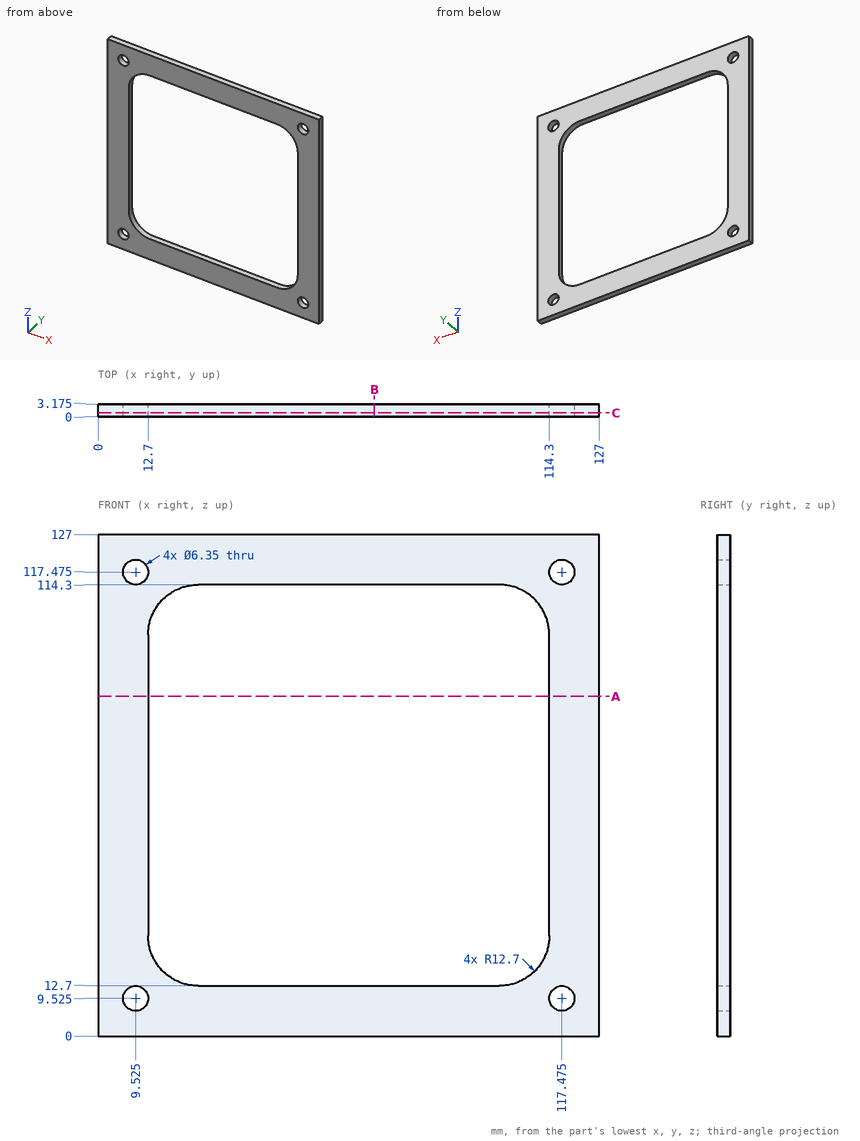
Geometry: see drawing. Coordinates: mm, zero at the bounding-box minimum. Coordinates: 2 decimals unless noted, no trailing zeros. Loops run counter-clockwise (first coordinate to the right, second up) from the corner with the lowest first, then second, coordinate; pieces in that order, holes last. Notation, with made-up numbers: M 6.25,45.25 L 12.25,45.25 A16 ccw 12.25,57.25 Z; hole C -13,54 d11. An arc over 180 degrees is marked long. Put each result on its own line as item: value. Start each with the question number.
1) Cut plane B-B on x = 70. Return the cut outline in (y, z) (3 decimals).
2) Cut plane C-C on y = 0.9. Return the cut outline in (x, z) (3 decimals).
3) Ray query, L1, parallel to Z at x = 36, y = 2.05; L2, parallel to Z at x = 118.5, y = 1.1. Return the intervals inside material, ascending. Write a range as from..to.
4) Cut plane A-A on z = 86. Return the cut outline in (x, y) (3 decimals), then the cut area to 3 significant figures.
The answers:
1. outline: M 0,0 L 3.175,0 L 3.175,12.7 L 0,12.7 Z; M 0,114.3 L 3.175,114.3 L 3.175,127 L 0,127 Z
2. outline: M 0,0 L 127,0 L 127,127 L 0,127 Z; hole C 9.525,9.525 d6.35; hole C 9.525,117.475 d6.35; hole M 12.7,25.4 A12.7 ccw 25.4,12.7 L 101.6,12.7 A12.7 ccw 114.3,25.4 L 114.3,101.6 A12.7 ccw 101.6,114.3 L 25.4,114.3 A12.7 ccw 12.7,101.6 Z; hole C 117.475,9.525 d6.35; hole C 117.475,117.475 d6.35
3. L1: z = 0..12.7, 114.3..127
3. L2: z = 0..6.52, 12.53..114.47, 120.48..127
4. outline: M 0,0 L 12.7,0 L 12.7,3.175 L 0,3.175 Z; M 114.3,0 L 127,0 L 127,3.175 L 114.3,3.175 Z
4. area: 80.6 mm²
